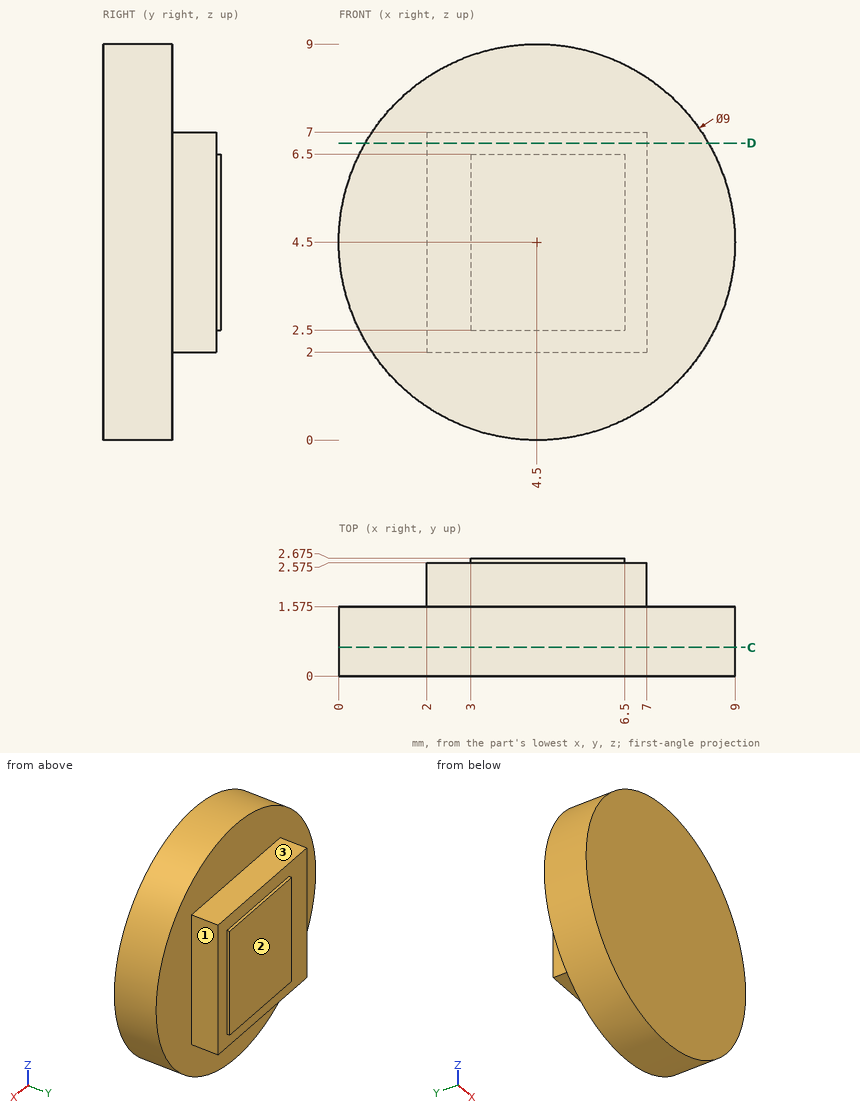
Geometry: see drawing. Coordinates: mm, zero at the bounding-box minimum. A direction names the side the tool comes from. Round coordinates to 2 decimals unless told otherwise and drop trailing zeros. Loops run counter-clockwise (first coordinate to the right, second up) from the corner with the lowest first, then second, coordinate; pieces in that order, holes last. Notation, with made-up numbers: M 87.25,89 L 98.25,89 A24 cw 98.25,102 Z; hole C 20,-2.75 d5. An arc over 180 degrees is marked long. Use a Markdown table: item, result. Add a question column.
1. Cut plane D-D, the plane z = 6.75. Output: boundary loops of the cut face in (x, y) (1 decimal).
2. Cut plane C-C, the plane y = 0.65. Output: boundary loops of the cut face in (x, z), and give its area (3 significant figures).
3. Contact query for flat-ended pins moving along their axis: pin 1 (1.1 mm diameter, centred on x = 5.5, y = 2, fed in from -Z); pin 2 (0.5 mm diameter, centred on y = 2.5, z = 5.5, fed in from +X); pin 3 (1 mm diameter, centred on x = 2.5, y = 2, fed in from -Z). Output: stop coordinate, or through.
4. Ray query, line 1 along Y through (x, z) = (1.5, 5.5) (1 decimal); line 2 along X through (y, z) = (2.35, 2.5). Return the intervals inside material, ascending. Write a range as [from, to].
5. Set-up query: the marked faces 1, 2 and 3. Return all of +Z, -Z, +X, -X, +Y, -Y with unobstructed straight access to the full face (end or side cutting, diameter ignored); none if empty.
Solution:
| question | item | result |
|---|---|---|
| 1 | outline | M 0.6,0 L 8.4,0 L 8.4,1.6 L 7,1.6 L 7,2.6 L 2,2.6 L 2,1.6 L 0.6,1.6 Z |
| 2 | outline | C 4.5,4.5 d9 |
| 2 | area | 63.6 mm2 |
| 3 | pin 1 | stops at z = 0.05 |
| 3 | pin 2 | stops at x = 7 |
| 3 | pin 3 | stops at z = 0.35 |
| 4 | line 1 | y = [0, 1.6] |
| 4 | line 2 | x = [2, 7] |
| 5 | face 1 | +Z, -Z, +X, +Y |
| 5 | face 2 | +Z, -Z, +X, -X, +Y |
| 5 | face 3 | +Z, +X, -X, +Y |
